Can you work these out from the model? Positions are in its coordinate system, mm. Face numbers are marked on the shaded views. A direction names the side the tool comes from. Give positions to 0.01 mm unless a question says otherwise; leave off trailing zeros. Write each loop counter-clockwise with the first axis right and the second up, starting at its lowest first coordinate (ties: lowest second). Pieces come first, ordered by that corner, then holes. Notation, with made-up numbers: M -34,-6 L 16,-6 A26 cw 16,22 Z; hole C -38.5,57.25 d9. An arc over 180 degrees is marked long. Write each question's results on one line, items separated by ' | '.
from build123d import *

# Parameters (mm, degrees)
BASE_DEPTH           = 12
BASE_DEPTH_BACK      = 5
ESQUISSE1_R          = 40
VIDE_PNEU_DEPTH      = 9
VIDE_PNEU_DEPTH_BACK = 2
ESQUISSE4_R          = 40
ESQUISSE4_R_2        = 37


with BuildPart() as part:
    # Esquisse1 → BASE (new, two sides: drawn at the far end of the back side and taken through both)
    with BuildSketch(Plane(origin=(0, 0, 0), x_dir=(0, 0, -1), z_dir=(1, 0, 0)).offset(-BASE_DEPTH_BACK)):
        Circle(ESQUISSE1_R)
        with BuildLine():
            Line((-1.658312395, 2.5), (1.658312395, 2.5))
            ThreePointArc((1.658312395, 2.5), (0, -3), (-1.658312395, 2.5))
        make_face(mode=Mode.SUBTRACT)
    extrude(amount=BASE_DEPTH + BASE_DEPTH_BACK)

    # Esquisse4 → VIDE PNEU (cut, two sides: drawn at the far end of the back side and taken through both)
    with BuildSketch(Plane(origin=(0, 0, 0), x_dir=(0, 0, -1), z_dir=(1, 0, 0)).offset(-VIDE_PNEU_DEPTH_BACK)):
        Circle(ESQUISSE4_R)
        Circle(ESQUISSE4_R_2, mode=Mode.SUBTRACT)
    extrude(amount=VIDE_PNEU_DEPTH + VIDE_PNEU_DEPTH_BACK, mode=Mode.SUBTRACT)


solid = part.part
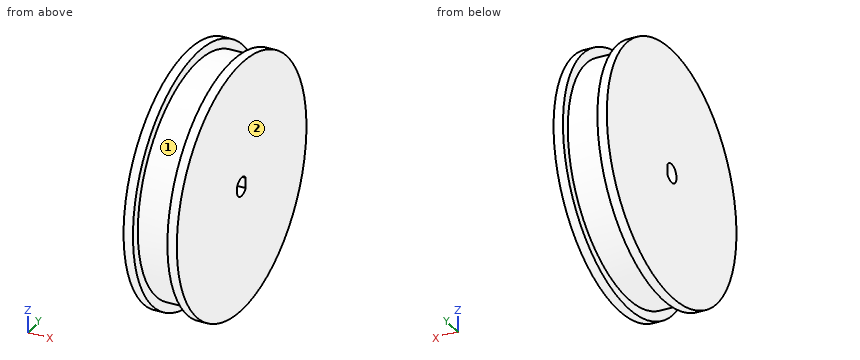
Item 1: I want a section at B-B, the plane z = 0. Please give me the cut outline in (x, y), and give its area (3 significant figures).
Geometry says:
outline: M -5,-40 L -2,-40 L -2,-37 L 9,-37 L 9,-40 L 12,-40 L 12,-3 L -5,-3 Z; M -5,2.5 L 12,2.5 L 12,40 L 9,40 L 9,37 L -2,37 L -2,40 L -5,40 Z | area: 1,200 mm2
Item 2: If I drill on line 1 (Y direction, x = 4, z = 0); line 2 (Y direction, x = -1, z = 1.5); line 3 (Z direction, x = 3, y = 2), over which ranges is the centre line in solid material (lowest first)? Write a range as from..to.
Geometry says:
line 1: y = -37..-3, 2.5..37 | line 2: y = -36.97..-2.6, 2.5..36.97 | line 3: z = -36.95..-2.24, 2.24..36.95
Item 3: I want a section at C-C, the plane x = 7. Please give me the cut outline in (y, z).
Geometry says:
outline: C 0,0 d74; hole M 2.5,-1.66 L 2.5,1.66 A3 ccw long Z
Item 4: I want a section at A-A, the plane y = 0. Please give me the cut outline in (x, z), and give its area (3 significant figures).
Geometry says:
outline: M -5,-40 L -2,-40 L -2,-37 L 9,-37 L 9,-40 L 12,-40 L 12,-3 L -5,-3 Z; M -5,3 L 12,3 L 12,40 L 9,40 L 9,37 L -2,37 L -2,40 L -5,40 Z | area: 1,190 mm2
Item 5: For the marked faces 1 and 2, which set-ups out of +Z, -Z, +X, -X, +Y, -Y let a thin tool reach every point of the face, with its end or its side?
Geometry says:
face 1: none | face 2: +Z, -Z, +X, +Y, -Y
Item 6: I'm going to push flat-ended pins straight in: pin 1 (4 mm diameter, centred on x = 8, z = 11.5, fed in from -Y); pin 2 (5.5 mm diameter, centred on y = 0, z = 0, fed in from -X); pin 3 (2.5 mm diameter, centred on x = 1.5, z = 0.5, fed in from -Y); pin 4 (6 mm diameter, centred on x = 3.5, z = -15.5, fed in from +Y). Where does each tip first touch, or does it pass through?
Geometry says:
pin 1: stops at y = -38.79 | pin 2: stops at x = -5 | pin 3: stops at y = -37 | pin 4: stops at y = 34.82
Item 7: I want a section at D-D, the plane y = 10. Please give me the cut outline in (x, z).
Geometry says:
outline: M -5,-38.73 L -2,-38.73 L -2,-35.62 L 9,-35.62 L 9,-38.73 L 12,-38.73 L 12,38.73 L 9,38.73 L 9,35.62 L -2,35.62 L -2,38.73 L -5,38.73 Z
